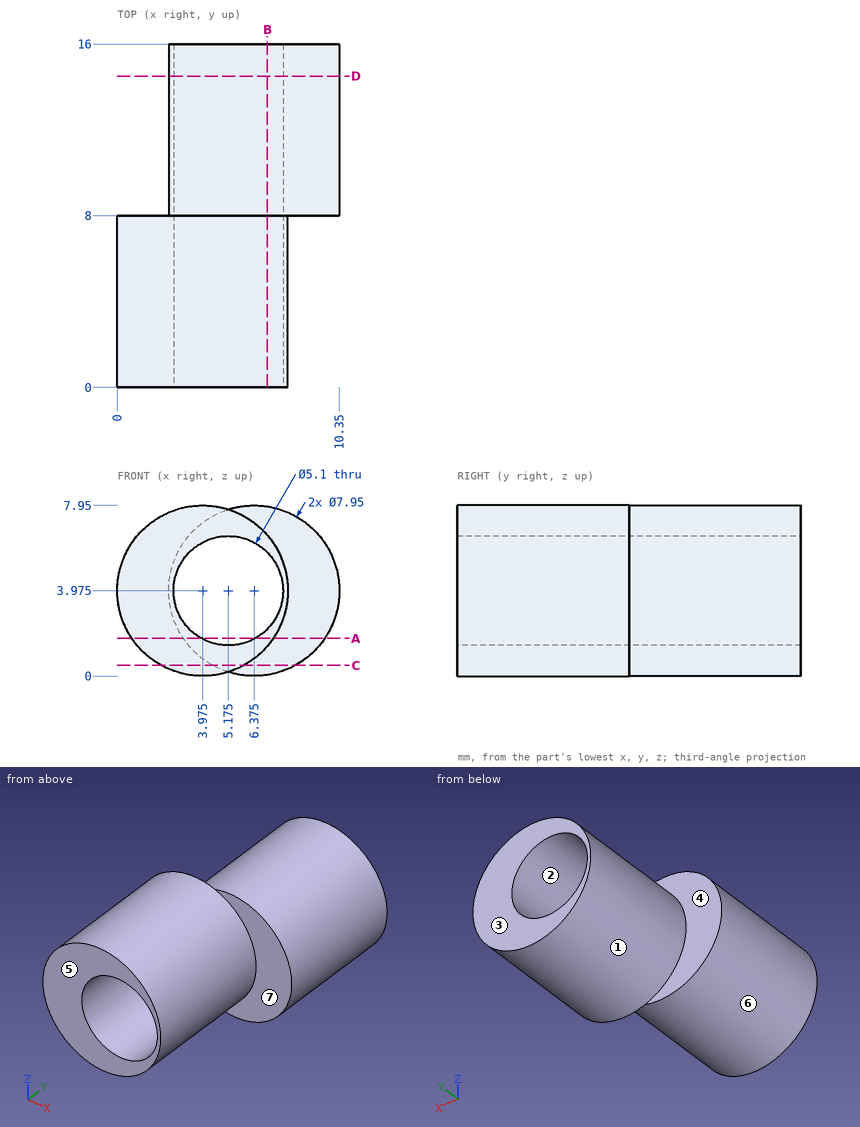
Job drawing, mm, ordinate dimensions from the low corner. One solid piece. A direction names the side the tool comes from. Coordinates: 2 decimals unless noted, no trailing zeros. Write each loop counter-clockwise with the first axis right and the second up, starting at its lowest first coordinate (ties: lowest second). Pieces come first, ordered by that corner, then holes.
Item 1: Slice it at B-B (x = 7). Write the cut outline in (y, z).
Item 2: Probe line 1 (X direction, y = 14.75, z = 2.5); line 2 (X direction, y = 5.25, z = 3); line 3 (Z direction, x = 6.5, y = 12). List the from-to ranges inside material, lowest first.
Item 3: Mould opens along Z. For the marked faces 1, 2 and 3 say: released by +Z, released by -Z, zero draft, split by the parting line, or undercut.
Item 4: Which spindle directions (+Z, -Z, +X, -X, +Y, -Y) get a long thin tool onto all of the face, cutting with end or side? Do the marked faces 4, 5, 6 and 7. Say none if no direction does.
Item 5: Pin check, flat tips, straight feed: pin 1 (1.5 mm diameter, centred on x = 3, y = 8, fed in from +Z); pin 2 (3 mm diameter, centred on y = 12, z = 7, fed in from -X); pin 3 (3 mm diameter, centred on y = 11, z = 6.5, fed in from -X). Stop position of each tip, or through.
Item 6: Slice it at C-C (z = 0.5). Write the cut outline in (x, y).
Item 7: Slice it at A-A (z = 1.75). Write the cut outline in (x, y).
Item 8: Slice it at D-D (y = 14.5). Write the cut outline in (x, z) (3 decimals).
Results found:
1. outline: (0, 1.4) - (8, 1.4) - (8, 0.05) - (16, 0.05) - (16, 2.19) - (0, 2.19) - close; (0, 5.76) - (16, 5.76) - (16, 7.9) - (8, 7.9) - (8, 6.55) - (0, 6.55) - close
2. line 1: x = 2.68 to 3.09, 7.26 to 10.07
2. line 2: x = 0.12 to 2.82, 7.53 to 7.83
2. line 3: z = 0 to 1.8, 6.15 to 7.95
3. face 1: split by the parting line
3. face 2: undercut
3. face 3: zero draft
4. face 4: -X, +Y
4. face 5: +Z, -Z, +X, -X, -Y
4. face 6: -Y
4. face 7: +X, -Y
5. pin 1: stops at z = 7.94
5. pin 2: stops at x = 2.7
5. pin 3: stops at x = 2.53
6. outline: (2.04, 0) - (5.91, 0) - (5.91, 8) - (8.31, 8) - (8.31, 16) - (4.44, 16) - (4.44, 8) - (2.04, 8) - close
7. outline: (0.68, 0) - (3.93, 0) - (3.93, 16) - (3.08, 16) - (3.08, 8) - (0.68, 8) - close; (6.42, 0) - (7.27, 0) - (7.27, 8) - (9.67, 8) - (9.67, 16) - (6.42, 16) - close
8. outline: circle Ø7.95 at (6.375, 3.975); hole circle Ø5.1 at (5.175, 3.975)
